Geometry check sheet. Reference: the model listing, model coordinates, mm. A direction names the side the tool comes from. Coordinates: 2 decimals unless noted, no trailing zeros. Order: outer loops, then holes, each group sorted by start corner. A loop starts at its lowest first (then second) coordinate and runs counter-clockwise, first axis right, second up. Notation, with made-up numbers: (-21, -27.75) -> (25, -27.75) arc R35 cw to (25, 8.25) -> close; hole circle Ø10 at (72, 59.5). An arc over 180 degrees is marked (long way). Answer in a Markdown table with one row per item. Add a question column.
```python
from build123d import *

# Parameters (mm, degrees)
SKETCH1_W           = 25
SKETCH1_H           = 25
BOSS_EXTRUDE1_DEPTH = 2
SKETCH2_R           = 1.15
CUT_EXTRUDE1_DEPTH  = 2
CUT_EXTRUDE2_DEPTH  = 1
FILLET1_R           = 1


with BuildPart() as part:
    # Sketch1 → Boss-Extrude1 (new body)
    with BuildSketch(Plane(origin=(0, 0, 0), x_dir=(1, 0, 0), z_dir=(0, 1, 0))):
        Rectangle(SKETCH1_W, SKETCH1_H)
    extrude(amount=BOSS_EXTRUDE1_DEPTH)

    # Sketch2 → Cut-Extrude1 (cut)
    with BuildSketch(Plane(origin=(0, 2, 0), x_dir=(1, 0, 0), z_dir=(0, 1, 0))):
        with Locations(Location((-8.5, 8.5, 0), (0, 0, 270))):
            Circle(SKETCH2_R)
        with Locations(Location((-8.5, -8.5, 0), (0, 0, 90))):
            Circle(SKETCH2_R)
        with Locations(Location((8.5, -8.5, 0), (0, 0, 270))):
            Circle(SKETCH2_R)
        with Locations(Location((8.5, 8.5, 0), (0, 0, 90))):
            Circle(SKETCH2_R)
    extrude(amount=-CUT_EXTRUDE1_DEPTH, mode=Mode.SUBTRACT)

    # Sketch3 → Cut-Extrude2 (cut)
    with BuildSketch(Plane(origin=(0, 2, 0), x_dir=(1, 0, 0), z_dir=(0, 1, 0))):
        with BuildLine():
            Line((10.675, -11.675), (-10.675, -11.675))
            ThreePointArc((-10.675, -11.675), (-11.382106781, -11.382106781), (-11.675, -10.675))
            Line((-11.675, -10.675), (-11.675, 10.675))
            ThreePointArc((-11.675, 10.675), (-11.382106781, 11.382106781), (-10.675, 11.675))
            Line((-10.675, 11.675), (10.675, 11.675))
            ThreePointArc((10.675, 11.675), (11.382106781, 11.382106781), (11.675, 10.675))
            Line((11.675, 10.675), (11.675, -10.675))
            ThreePointArc((11.675, -10.675), (11.382106781, -11.382106781), (10.675, -11.675))
        make_face()
    extrude(amount=-CUT_EXTRUDE2_DEPTH, mode=Mode.SUBTRACT)

    # Fillet1
    fillet1_edges = [part.edges().sort_by_distance(p)[0] for p in [
        (12.5, 1, 12.5),
        (-12.5, 1, 12.5),
        (-12.5, 1, -12.5),
        (12.5, 1, -12.5),
    ]]
    fillet(fillet1_edges, radius=FILLET1_R)


solid = part.part
```
(1) Cross-section at A-A (x = -8.5). Enter the section's corners in (y, z) (3 decimals).
(2) Go/stop test with flat-tipped pins: P1, Ø11.5, axis at x = -6, z = -4, coming from the +Y side; P2, Ø2, axis at x = 8.5, z = 8.5, coming from the +Y side; P3, Ø5, axis at x = -5, z = -9, coming from the +Y side. Record where each tip stops, or that it passes through.
(3) Cross-section at B-B (y = 0.6). Enter the section's corners in (x, z), plus the area to 3 significant figures.
(4) Access from +Z, -Z, +X, -X, +Y, -Y to the whole of each face (thin tool, end or side, straight path). Record for faces 1 (the face through (12.199, 1.014, -12.215)), 2 (the face through (11.39, 1.507, 11.374)).
(5) Mould release check, pull along X, two halves, no side actions. Record for faces 3 (the face through (11.675, 1.5, -0.1)), 4 (the face through (12.199, 1.014, 12.215)), 5 (the face through (-1, 2, 12)), 6 (the face through (8.94, 0.507, -9.562)): +X half, -X half, draft (parallel to the pull), parting line (faces both ways), or undercut.
(6) Cross-section at C-C (z = 8.5). Enter the section's corners in (x, y) (3 decimals), plus the area to 4 significant figures.
(7) Scan lines: line 1 along X through (y, z) = (0.35, 8.5); line 2 along X through (y, z) = (1.35, 4) (3 decimals). Record each from-to range of solid material in increasing order.
(8) Cross-section at D-D (z = 0.75). Enter the section's corners in (x, y) (3 decimals).
Checks:
| question | item | result |
|---|---|---|
| 1 | outline | (0, -12.5) -> (2, -12.5) -> (2, -11.675) -> (1, -11.675) -> (1, -9.65) -> (0, -9.65) -> close; (0, -7.35) -> (1, -7.35) -> (1, 7.35) -> (0, 7.35) -> close; (0, 9.65) -> (1, 9.65) -> (1, 11.675) -> (2, 11.675) -> (2, 12.5) -> (0, 12.5) -> close |
| 2 | P1 | y = 2 |
| 2 | P2 | through |
| 2 | P3 | y = 1 |
| 3 | outline | (-12.5, -11.5) arc R1 ccw to (-11.5, -12.5) -> (11.5, -12.5) arc R1 ccw to (12.5, -11.5) -> (12.5, 11.5) arc R1 ccw to (11.5, 12.5) -> (-11.5, 12.5) arc R1 ccw to (-12.5, 11.5) -> close; hole circle Ø2.3 at (-8.5, -8.5); hole circle Ø2.3 at (-8.5, 8.5); hole circle Ø2.3 at (8.5, -8.5); hole circle Ø2.3 at (8.5, 8.5) |
| 3 | area | 608 mm² |
| 4 | face 1 | -Z, +X, +Y, -Y |
| 4 | face 2 | +Y |
| 5 | face 3 | undercut |
| 5 | face 4 | +X half |
| 5 | face 5 | draft |
| 5 | face 6 | undercut |
| 6 | outline | (-12.5, 0) -> (-9.65, 0) -> (-9.65, 1) -> (-11.675, 1) -> (-11.675, 2) -> (-12.5, 2) -> close; (-7.35, 0) -> (7.35, 0) -> (7.35, 1) -> (-7.35, 1) -> close; (9.65, 0) -> (12.5, 0) -> (12.5, 2) -> (11.675, 2) -> (11.675, 1) -> (9.65, 1) -> close |
| 6 | area | 22.05 mm² |
| 7 | line 1 | -12.5 to -9.65, -7.35 to 7.35, 9.65 to 12.5 |
| 7 | line 2 | -12.5 to -11.675, 11.675 to 12.5 |
| 8 | outline | (-12.5, 0) -> (12.5, 0) -> (12.5, 2) -> (11.675, 2) -> (11.675, 1) -> (-11.675, 1) -> (-11.675, 2) -> (-12.5, 2) -> close |
